CAD build for the part. Positions are in the model's coordinates, mm. A direction names the side the tool comes from. Give positions to 0.01 mm unless a question says otherwise; leave off trailing zeros. Write each loop counter-clockwise with the first axis right and the second up, starting at its lowest first coordinate (ties: lowest second). Pieces come first, ordered by that corner, then holes. Notation, with made-up numbers: M -19.5,-16.75 L 16.5,-16.75 A29 ccw 16.5,6.25 Z; hole C -5.5,81.5 d8. An arc over 180 degrees is marked long. One line per question, with ' | ' between items. Start each with the question number.
1. Cut at B-B, the plane z = 2.05. Write the cut outline in (x, y) (3 decimals).
2. Pull direction Y, two halves, no side cores. Call faces 3 (the face through (-9, -15.275, 1)), 4 (the face through (10, -15.275, 1)), 5 (the face through (-3, -20, 1.3)): released by +Y, released by -Y, zero draft, split by the parting line, or undercut.
3. Flat gauge pins, fed straight in: pin 1 (1 mm diameter, centred on x = -19.5, y = -12, fed in from +Z); pin 2 (1 mm diameter, centred on y = 8.5, z = 2, fed in from +X) (3 decimals); pin 3 (0.6 mm diameter, centred on y = 8.5, z = 2, fed in from -X) (3 decimals). Where does each tip first touch, or does it go through?
4. Cut at C-C, the plane y = -2. Write the cut outline in (x, z) (3 decimals).
5. Cut at D-D, the plane x = -0.5. Write the cut outline in (y, z) (3 decimals).
6. Which spindle directions (+Z, -Z, +X, -X, +Y, -Y) get a long thin tool onto all of the face, cutting with end or side? Do faces 1 (the face through (32.025, -8, 1)), 2 (the face through (-1, 0, 2.5)). Say none if no direction does.
7. Wall check: L1, parallel to Y at x = 22, z = 2.25 (3 decimals); L2, parallel to X at y = -8.5, z = 0.7 (3 decimals); L3, parallel to Y at x = -14.5, z = 0.8 (3 decimals). Give the ranges that are in metal, low to high.
8. Cut at A-A, the plane x = -30.1. Write the cut outline in (y, z) (3 decimals), then the cut area to 3 significant figures.
```python
from build123d import *

# Parameters (mm, degrees)
F0_W     = 79.85
F0_H     = 38.55
F0_R     = 4.25
F0_W_2   = 12.7
F0_H_2   = 15
F0_R_2   = 2.75
F1_DEPTH = 2.5
F0_W_3   = 83.65
F0_H_3   = 42.35
F2_DEPTH = 1.3


with BuildPart() as f1:
    # F0 (on Top) → F1 (new body)
    with BuildSketch(Plane.XY):
        Rectangle(F0_W, F0_H)
        with Locations((-30.1, -0.275)):
            Circle(F0_R, mode=Mode.SUBTRACT)
        Polygon((1.025, -6.275), (1.025, -15.275), (-20.275, -15.275), (-20.275, -6.275), (-16.925, -6.275), (-16.925, -4.075), (-14.425, -4.075), (-14.425, -6.275), (-6.275, -6.275), (-6.275, -4.075), (-3.775, -4.075), (-3.775, -6.275), align=None, mode=Mode.SUBTRACT)
        with Locations((9.675, -7.775)):
            Rectangle(F0_W_2, F0_H_2, mode=Mode.SUBTRACT)
        with Locations((25.675, -7.775)):
            Rectangle(F0_W_2, F0_H_2, mode=Mode.SUBTRACT)
        with Locations((-9.625, 11.775)):
            Circle(F0_R_2, mode=Mode.SUBTRACT)
        with Locations((9.675, 11.775)):
            Circle(F0_R_2, mode=Mode.SUBTRACT)
        with Locations((25.675, 11.775)):
            Circle(F0_R_2, mode=Mode.SUBTRACT)
    extrude(amount=F1_DEPTH)

    # F0 (on Top) → F2 (join)
    with BuildSketch(Plane.XY):
        Rectangle(F0_W_3, F0_H_3)
        Rectangle(F0_W, F0_H, mode=Mode.SUBTRACT)
    extrude(amount=F2_DEPTH)


solid = f1.part
```
Here are the results:
1) outline: M -39.925,-19.275 L 39.925,-19.275 L 39.925,19.275 L -39.925,19.275 Z; hole C -30.1,-0.275 d8.5; hole M -20.275,-15.275 L 1.025,-15.275 L 1.025,-6.275 L -3.775,-6.275 L -3.775,-4.075 L -6.275,-4.075 L -6.275,-6.275 L -14.425,-6.275 L -14.425,-4.075 L -16.925,-4.075 L -16.925,-6.275 L -20.275,-6.275 Z; hole C -9.625,11.775 d5.5; hole M 3.325,-15.275 L 16.025,-15.275 L 16.025,-0.275 L 3.325,-0.275 Z; hole C 9.675,11.775 d5.5; hole M 19.325,-15.275 L 32.025,-15.275 L 32.025,-0.275 L 19.325,-0.275 Z; hole C 25.675,11.775 d5.5
2) face 3: undercut | face 4: undercut | face 5: zero draft
3) pin 1: through | pin 2: x = 39.925 | pin 3: x = -39.925
4) outline: M -41.825,0 L -33.984,0 L -33.984,2.5 L -39.925,2.5 L -39.925,1.3 L -41.825,1.3 Z; M -26.216,0 L 3.325,0 L 3.325,2.5 L -26.216,2.5 Z; M 16.025,0 L 19.325,0 L 19.325,2.5 L 16.025,2.5 Z; M 32.025,0 L 41.825,0 L 41.825,1.3 L 39.925,1.3 L 39.925,2.5 L 32.025,2.5 Z
5) outline: M -21.175,0 L -15.275,0 L -15.275,2.5 L -19.275,2.5 L -19.275,1.3 L -21.175,1.3 Z; M -6.275,0 L 21.175,0 L 21.175,1.3 L 19.275,1.3 L 19.275,2.5 L -6.275,2.5 Z
6) face 1: +Z, -Z | face 2: +Z, +X, -X, +Y, -Y
7) L1: -19.275 to -15.275, -0.275 to 19.275 | L2: -41.825 to -20.275, 1.025 to 3.325, 16.025 to 19.325, 32.025 to 41.825 | L3: -21.175 to -15.275, -4.075 to 21.175
8) outline: M -21.175,0 L -4.525,0 L -4.525,2.5 L -19.275,2.5 L -19.275,1.3 L -21.175,1.3 Z; M 3.975,0 L 21.175,0 L 21.175,1.3 L 19.275,1.3 L 19.275,2.5 L 3.975,2.5 Z | area: 80.1 mm^2
